Verification items for the finished model (mm, model axes). A direction names the side the tool comes from. Give positions to 0.01 mm unless a question says otherwise; leave off trailing zeros. Loops run counter-clockwise (first coordinate to the right, second up) from the corner with the lowest first, then second, coordinate; pieces in that order, holes last. Notation, with made-up numbers: (-11, 76) -> (27, 76) arc R33 cw to (27, 113) -> close; hole circle Ø5 at (6.25, 41.25). An arc over 180 degrees is marked (long way). Use one line per item in the form item = value. Start each with the question number.
from build123d import *

# Parameters (mm, degrees)
F0_W     = 101.6
F0_H     = 76.2
F1_DEPTH = 25.4
F2_R     = 25.4
F3_DEPTH = 25.4
F4_R     = 15.24
F5_DEPTH = 61.722


with BuildPart() as f1:
    # F0 (on Front) → F1 (new body)
    with BuildSketch(Plane.XZ):
        Rectangle(F0_W, F0_H)
    extrude(amount=F1_DEPTH)

    # F2 (on face) → F3 (join)
    with BuildSketch(Plane.XZ.offset(25.4)):
        Circle(F2_R)
    extrude(amount=F3_DEPTH)

    # F4 (on face) → F5 (cut)
    with BuildSketch(Plane.XZ.offset(50.8)):
        Circle(F4_R)
    extrude(amount=-F5_DEPTH, mode=Mode.SUBTRACT)


solid = f1.part
Item 1: Sectioned sample at D-D, the plane z = -21.5. Enter the section's corners in (x, y), and give its area (3 significant figures).
Item 2: Sectioned sample at B-B, the plane y = -18. Enter the section's corners in (x, z).
Item 3: Gauge pin test, flat ends, axial feed: pin 1 Ø5 at (x, z) = (-32.5, 26) entering from -Y; pin 2 Ø2 at (y, z) = (-35.5, 12.5) entering from +X; pin 3 Ø3 at (x, y) = (12.5, -34) entering from +Z. Record the tip position at first contact, or that the pin passes through.
Item 4: Tool access check on faces 4 (the flat face through (-1, -25.4, 26)), 5 (the flat face through (-1, 0, 17)). Record the directions out of +Z, -Z, +X, -X, +Y, -Y that give a thin tool (end or side, any length) a straight path to the whole face; none if there is none.
Item 5: Sectioned sample at A-A, the plane z = 0. Enter the section's corners in (x, y), and give its area (3 significant figures).
Item 6: Material ranges on line 1 (X direction, y = -21, z = -0.5); line 2 (Z direction, x = 0, y = -35); line 3 (Z direction, x = 0, y = -25), recorded low to high.
Item 7: Sectioned sample at C-C, the plane x = -11. Enter the section's corners in (y, z), and give its area (3 significant figures).
Item 8: Draft check along Z on faces 1 (the flat face through (-1, -13, -38.1)), 2 (the cylindrical face through (-3.3, -25.76, -14.88)), 3 (the flat face through (-50.8, -13, -1)). Enter one of: +Z half, -Z half, draft (parallel to the pull), parting line (faces both ways), or undercut.
Outcome:
q1.outline = (-50.8, -25.4) -> (-13.52, -25.4) -> (-13.52, -50.8) -> (13.52, -50.8) -> (13.52, -25.4) -> (50.8, -25.4) -> (50.8, 0) -> (-50.8, 0) -> close
q1.area = 3,270 mm^2
q2.outline = (-50.8, -38.1) -> (50.8, -38.1) -> (50.8, 38.1) -> (-50.8, 38.1) -> close; hole circle Ø30.48 at (0, 0)
q3.pin_1 = -25.4
q3.pin_2 = 22.65
q3.pin_3 = 22.89
q4.face_4 = -Y
q4.face_5 = +Z, -Z, +X, -X, +Y
q5.outline = (-50.8, -25.4) -> (-25.4, -25.4) -> (-25.4, -50.8) -> (-15.24, -50.8) -> (-15.24, 0) -> (-50.8, 0) -> close; (15.24, -50.8) -> (25.4, -50.8) -> (25.4, -25.4) -> (50.8, -25.4) -> (50.8, 0) -> (15.24, 0) -> close
q5.area = 2,320 mm^2
q6.line_1 = -50.8 to -15.23, 15.23 to 50.8
q6.line_2 = -25.4 to -15.24, 15.24 to 25.4
q6.line_3 = -38.1 to -15.24, 15.24 to 38.1
q7.outline = (-50.8, -22.89) -> (-25.4, -22.89) -> (-25.4, -38.1) -> (0, -38.1) -> (0, -10.55) -> (-50.8, -10.55) -> close; (-50.8, 10.55) -> (0, 10.55) -> (0, 38.1) -> (-25.4, 38.1) -> (-25.4, 22.89) -> (-50.8, 22.89) -> close
q7.area = 2,030 mm^2
q8.face_1 = -Z half
q8.face_2 = undercut
q8.face_3 = draft
